Input: part model. Units: mm. Frame: model coordinates. Face numbers are marked on the shaded views. A direction names the side the tool comes from. Coordinates: 2 decimals unless noted, no trailing zeros. Order: outer loops, then holes, each group sorted by start corner. A loop starts at its lowest first (then second) coordinate and runs counter-clockwise, first axis right, second up. Notation, with made-up numbers: (12, 44) - (51, 44) arc R8 cw to (51, 56) - close; hole circle Ø3 at (7, 56). An arc over 180 degrees is marked (long way). Use a Markdown table: item, result. Add a question column.
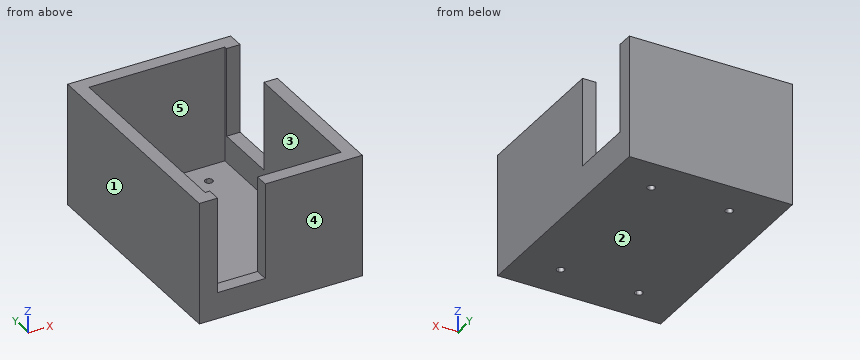
from build123d import *

# Parameters (mm, degrees)
F0_W     = 20.6896286374
F0_H     = 8.5261184722
F1_DEPTH = 45.72
F3_DEPTH = 43.18
F5_DEPTH = 25.4
F6_W     = 24.390142411
F6_H     = 33.248395839
F7_DEPTH = 25.4
F8_W     = 17.8320128471
F8_H     = 35.8616813955
F9_DEPTH = 25.4


with BuildPart() as f1:
    # F0 (on Top) → F1 (new body)
    with BuildSketch(Plane.XY):
        Polygon((36.2886708146, 54.0553010044), (-24.6713291854, 54.0553010044), (-24.6713291854, -32.0506989956), (15.5990421772, -32.0506989956), (15.5990421772, -23.5245805234), (36.2886708146, -23.5245805234), align=None)
        with Locations((25.9438564959, -27.7876397595)):
            Rectangle(F0_W, F0_H)
    extrude(amount=F1_DEPTH)

    # F2 (on face) → F3 (cut)
    with BuildSketch(Plane.XY.offset(45.72)):
        Polygon((5.8086708146, 48.9753010044), (-19.5913291854, 48.9753010044), (-19.5913291854, 11.0023010044), (-19.5913291854, -26.9706989956), (5.8086708146, -26.9706989956), (31.2086708146, -26.9706989956), (31.2086708146, 11.0023010044), (31.2086708146, 48.9753010044), align=None)
    extrude(amount=-F3_DEPTH, mode=Mode.SUBTRACT)

    # F4 (on face) → F5 (cut)
    with BuildSketch(Plane.XY.offset(2.54)):
        with BuildLine():
            Line((-8.7963291854, 40.5933010044), (-10.2568291854, 40.5933010044))
            ThreePointArc((-10.2568291854, 40.5933010044), (-9.8290586393, 39.5605715505), (-8.7963291854, 39.1328010044))
            Line((-8.7963291854, 39.1328010044), (-8.7963291854, 40.5933010044))
        make_face()
        with BuildLine():
            Line((-7.3358291854, 40.5933010044), (-8.7963291854, 40.5933010044))
            Line((-8.7963291854, 40.5933010044), (-8.7963291854, 39.1328010044))
            ThreePointArc((-8.7963291854, 39.1328010044), (-7.7635997314, 39.5605715505), (-7.3358291854, 40.5933010044))
        make_face()
        with BuildLine():
            ThreePointArc((-7.3358291854, 40.5933010044), (-7.7635997314, 41.6260304583), (-8.7963291854, 42.0538010044))
            Line((-8.7963291854, 42.0538010044), (-8.7963291854, 40.5933010044))
            Line((-8.7963291854, 40.5933010044), (-7.3358291854, 40.5933010044))
        make_face()
        with BuildLine():
            ThreePointArc((-8.7963291854, 42.0538010044), (-9.8290586393, 41.6260304583), (-10.2568291854, 40.5933010044))
            Line((-10.2568291854, 40.5933010044), (-8.7963291854, 40.5933010044))
            Line((-8.7963291854, 40.5933010044), (-8.7963291854, 42.0538010044))
        make_face()
        with BuildLine():
            Line((-8.7963291854, -17.1281989956), (-8.7963291854, -18.5886989956))
            Line((-8.7963291854, -18.5886989956), (-7.3358291854, -18.5886989956))
            ThreePointArc((-7.3358291854, -18.5886989956), (-7.7635997314, -17.5559695417), (-8.7963291854, -17.1281989956))
        make_face()
        with BuildLine():
            Line((-8.7963291854, -18.5886989956), (-10.2568291854, -18.5886989956))
            ThreePointArc((-10.2568291854, -18.5886989956), (-9.8290586393, -19.6214284495), (-8.7963291854, -20.0491989956))
            Line((-8.7963291854, -20.0491989956), (-8.7963291854, -18.5886989956))
        make_face()
        with BuildLine():
            Line((-7.3358291854, -18.5886989956), (-8.7963291854, -18.5886989956))
            Line((-8.7963291854, -18.5886989956), (-8.7963291854, -20.0491989956))
            ThreePointArc((-8.7963291854, -20.0491989956), (-7.7635997314, -19.6214284495), (-7.3358291854, -18.5886989956))
        make_face()
        with BuildLine():
            ThreePointArc((-8.7963291854, -17.1281989956), (-9.8290586393, -17.5559695417), (-10.2568291854, -18.5886989956))
            Line((-10.2568291854, -18.5886989956), (-8.7963291854, -18.5886989956))
            Line((-8.7963291854, -18.5886989956), (-8.7963291854, -17.1281989956))
        make_face()
        with BuildLine():
            ThreePointArc((21.8741708146, 40.5933010044), (21.4464002686, 41.6260304583), (20.4136708146, 42.0538010044))
            Line((20.4136708146, 42.0538010044), (20.4136708146, 40.5933010044))
            Line((20.4136708146, 40.5933010044), (21.8741708146, 40.5933010044))
        make_face()
        with BuildLine():
            Line((21.8741708146, 40.5933010044), (20.4136708146, 40.5933010044))
            Line((20.4136708146, 40.5933010044), (20.4136708146, 39.1328010044))
            ThreePointArc((20.4136708146, 39.1328010044), (21.4464002686, 39.5605715505), (21.8741708146, 40.5933010044))
        make_face()
        with BuildLine():
            Line((20.4136708146, 40.5933010044), (18.9531708146, 40.5933010044))
            ThreePointArc((18.9531708146, 40.5933010044), (19.3809413607, 39.5605715505), (20.4136708146, 39.1328010044))
            Line((20.4136708146, 39.1328010044), (20.4136708146, 40.5933010044))
        make_face()
        with BuildLine():
            Line((20.4136708146, 40.5933010044), (20.4136708146, 42.0538010044))
            ThreePointArc((20.4136708146, 42.0538010044), (19.3809413607, 41.6260304583), (18.9531708146, 40.5933010044))
            Line((18.9531708146, 40.5933010044), (20.4136708146, 40.5933010044))
        make_face()
        with BuildLine():
            ThreePointArc((21.8741708146, -18.5886989956), (21.4464002686, -17.5559695417), (20.4136708146, -17.1281989956))
            Line((20.4136708146, -17.1281989956), (20.4136708146, -18.5886989956))
            Line((20.4136708146, -18.5886989956), (21.8741708146, -18.5886989956))
        make_face()
        with BuildLine():
            ThreePointArc((20.4136708146, -17.1281989956), (19.3809413607, -17.5559695417), (18.9531708146, -18.5886989956))
            Line((18.9531708146, -18.5886989956), (20.4136708146, -18.5886989956))
            Line((20.4136708146, -18.5886989956), (20.4136708146, -17.1281989956))
        make_face()
        with BuildLine():
            ThreePointArc((18.9531708146, -18.5886989956), (19.3809413607, -19.6214284495), (20.4136708146, -20.0491989956))
            Line((20.4136708146, -20.0491989956), (20.4136708146, -18.5886989956))
            Line((20.4136708146, -18.5886989956), (18.9531708146, -18.5886989956))
        make_face()
        with BuildLine():
            Line((20.4136708146, -18.5886989956), (20.4136708146, -20.0491989956))
            ThreePointArc((20.4136708146, -20.0491989956), (21.4464002686, -19.6214284495), (21.8741708146, -18.5886989956))
            Line((21.8741708146, -18.5886989956), (20.4136708146, -18.5886989956))
        make_face()
    extrude(amount=-F5_DEPTH, mode=Mode.SUBTRACT)

    # F6 (on face) → F7 (cut)
    with BuildSketch(Plane.YZ.offset(36.2886708146)):
        with Locations((35.6818791479, 29.0958020805)):
            Rectangle(F6_W, F6_H)
    extrude(amount=-F7_DEPTH, mode=Mode.SUBTRACT)

    # F8 (on face) → F9 (cut)
    with BuildSketch(Plane.XZ.offset(32.0506989956)):
        with Locations((-8.9160064235, 27.7891593023)):
            Rectangle(F8_W, F8_H)
    extrude(amount=-F9_DEPTH, mode=Mode.SUBTRACT)


solid = f1.part
1) Pull-direction query (X, two-part tool) for the marked faces 1, 2 and 3; classes: pulls with the +X half, pulls with the -X half, needs draft (parallel to the pull), parting line crosses it, or undercut.
2) Material intervals for L1, parallel to X at y = 29, z = 9; L2, parallel to Y at x = -3, z = 6; L3, parallel to Y at x = 33.5, z = 38, sorted ascending.
3) Cut plane A-A (z = 35). Return the cut outline in (x, y), and give its area (3 significant figures).
4) Contact query for flat-ended pins moving along their axis: P1, Ø2, axis at x = 1.5, y = -5, coming from the +Z side; P2, Ø2.5, axis at x = -11, y = -28.5, coming from the +Z side; P3, Ø1.5, axis at x = 33.5, y = 39, coming from the +Z side. Output: stop coordinate, or through.
5) Cut plane B-B (x = 32.5). Return the cut outline in (y, z).
6) Cut plane C-C (y = -25). Return the cut outline in (x, z).
7) Reachability of the marked faces 4 and 5 from +Z, -Z, +X, -X, +Y, -Y: full face, straight path, thin tool, end or side. Return the list, or none.
Computed:
| question | item | result |
|---|---|---|
| 1 | face 1 | pulls with the -X half |
| 1 | face 2 | needs draft |
| 1 | face 3 | undercut |
| 2 | L1 | x = -24.67 to -19.59, 31.21 to 36.29 |
| 2 | L2 | y = -32.05 to -26.97, 48.98 to 54.06 |
| 2 | L3 | y = -32.05 to 23.49, 47.88 to 54.06 |
| 3 | outline | (-24.67, -32.05) - (-17.83, -32.05) - (-17.83, -26.97) - (-19.59, -26.97) - (-19.59, 48.98) - (31.21, 48.98) - (31.21, 47.88) - (36.29, 47.88) - (36.29, 54.06) - (-24.67, 54.06) - close; (0, -32.05) - (36.29, -32.05) - (36.29, 23.49) - (31.21, 23.49) - (31.21, -26.97) - (0, -26.97) - close |
| 3 | area | 1,180 mm2 |
| 4 | P1 | stops at z = 2.54 |
| 4 | P2 | stops at z = 9.86 |
| 4 | P3 | stops at z = 12.47 |
| 5 | outline | (-32.05, 0) - (54.06, 0) - (54.06, 45.72) - (47.88, 45.72) - (47.88, 12.47) - (23.49, 12.47) - (23.49, 45.72) - (-32.05, 45.72) - close |
| 6 | outline | (-24.67, 0) - (36.29, 0) - (36.29, 45.72) - (31.21, 45.72) - (31.21, 2.54) - (-19.59, 2.54) - (-19.59, 45.72) - (-24.67, 45.72) - close |
| 7 | face 4 | +Z, -Z, +X, -X, -Y |
| 7 | face 5 | +Z |
